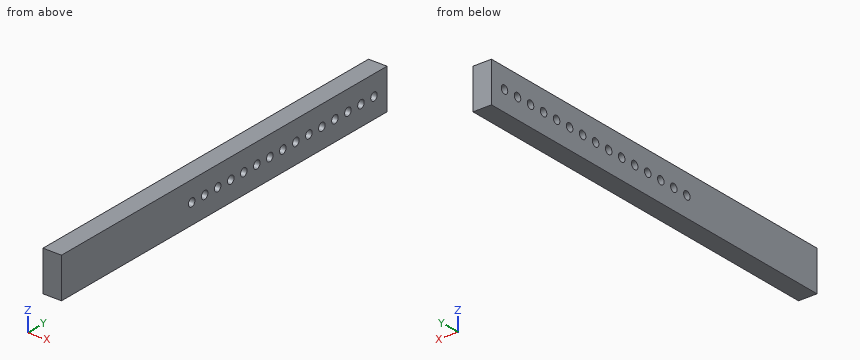
```python
from build123d import *

# Parameters (mm, degrees)
SKETCH1_W           = 50
SKETCH1_H           = 500
SKETCH1_R           = 5
BOSS_EXTRUDE1_DEPTH = 23


with BuildPart() as part:
    # Sketch1 → Boss-Extrude1 (new body)
    with BuildSketch(Plane(origin=(0, 0, 0), x_dir=(0, 0, -1), z_dir=(1, 0, 0))):
        Rectangle(SKETCH1_W, SKETCH1_H)
        with Locations((0, 230)):
            Circle(SKETCH1_R, mode=Mode.SUBTRACT)
        with Locations((0, 210)):
            Circle(SKETCH1_R, mode=Mode.SUBTRACT)
        with Locations((0, 190)):
            Circle(SKETCH1_R, mode=Mode.SUBTRACT)
        with Locations((0, 170)):
            Circle(SKETCH1_R, mode=Mode.SUBTRACT)
        with Locations((0, 150)):
            Circle(SKETCH1_R, mode=Mode.SUBTRACT)
        with Locations((0, 130)):
            Circle(SKETCH1_R, mode=Mode.SUBTRACT)
        with Locations((0, 110)):
            Circle(SKETCH1_R, mode=Mode.SUBTRACT)
        with Locations((0, 90)):
            Circle(SKETCH1_R, mode=Mode.SUBTRACT)
        with Locations((0, 70)):
            Circle(SKETCH1_R, mode=Mode.SUBTRACT)
        with Locations((0, 50)):
            Circle(SKETCH1_R, mode=Mode.SUBTRACT)
        with Locations((0, 30)):
            Circle(SKETCH1_R, mode=Mode.SUBTRACT)
        with Locations((0, 10)):
            Circle(SKETCH1_R, mode=Mode.SUBTRACT)
        with Locations((0, -10)):
            Circle(SKETCH1_R, mode=Mode.SUBTRACT)
        with Locations((0, -30)):
            Circle(SKETCH1_R, mode=Mode.SUBTRACT)
        with Locations((0, -50)):
            Circle(SKETCH1_R, mode=Mode.SUBTRACT)
    extrude(amount=BOSS_EXTRUDE1_DEPTH)


solid = part.part
```
Here's how the part is built. I have some questions about the finished solid (model axes, mm). Coordinates: 2 decimals unless noted, no trailing zeros. Loops run counter-clockwise (first coordinate to the right, second up) from the corner with the lowest first, then second, coordinate; pieces in that order, holes last. Notation, with made-up numbers: (-25.5, -16.75) - (2.5, -16.75) arc R20 ccw to (2.5, 0.25) - close; hole circle Ø1 at (35, 38.5). An arc over 180 degrees is marked (long way). Return JSON: item names as keys, results as strings. Group by question number.
Item 1: Will this pin go through, and if not, where does the flat tip stop? P1, Ø6, axis at y = 30, z = 0, coming from the -X side.
Item 2: I need wall thicknesses on line 1 (Z direction, x = 5.25, y = 111); line 2 (Z direction, x = 18.25, y = -32.5). Which ranges of each line are inside material? Lowest first, please. Write a range as from..to.
Item 3: If we section it at B-B on y = -50: Write out the boundary of the cut face in (x, z), and give its area (3 significant figures).
Item 4: If we section it at A-A on x = 11.75: State how many separate pieces and enclosed holes the cut face has, and give its area (3 significant figures).
Calculated:
{
 "1": {"P1": "passes through"},
 "2": {"line 1": "z = -25..-4.9, 4.9..25", "line 2": "z = -25..-4.33, 4.33..25"},
 "3": {"outline": "(0, -25) - (23, -25) - (23, -5) - (0, -5) - close; (0, 5) - (23, 5) - (23, 25) - (0, 25) - close", "area": "920 mm^2"},
 "4": {"separate pieces": "1", "enclosed holes": "15", "area": "23,800 mm^2"}
}
